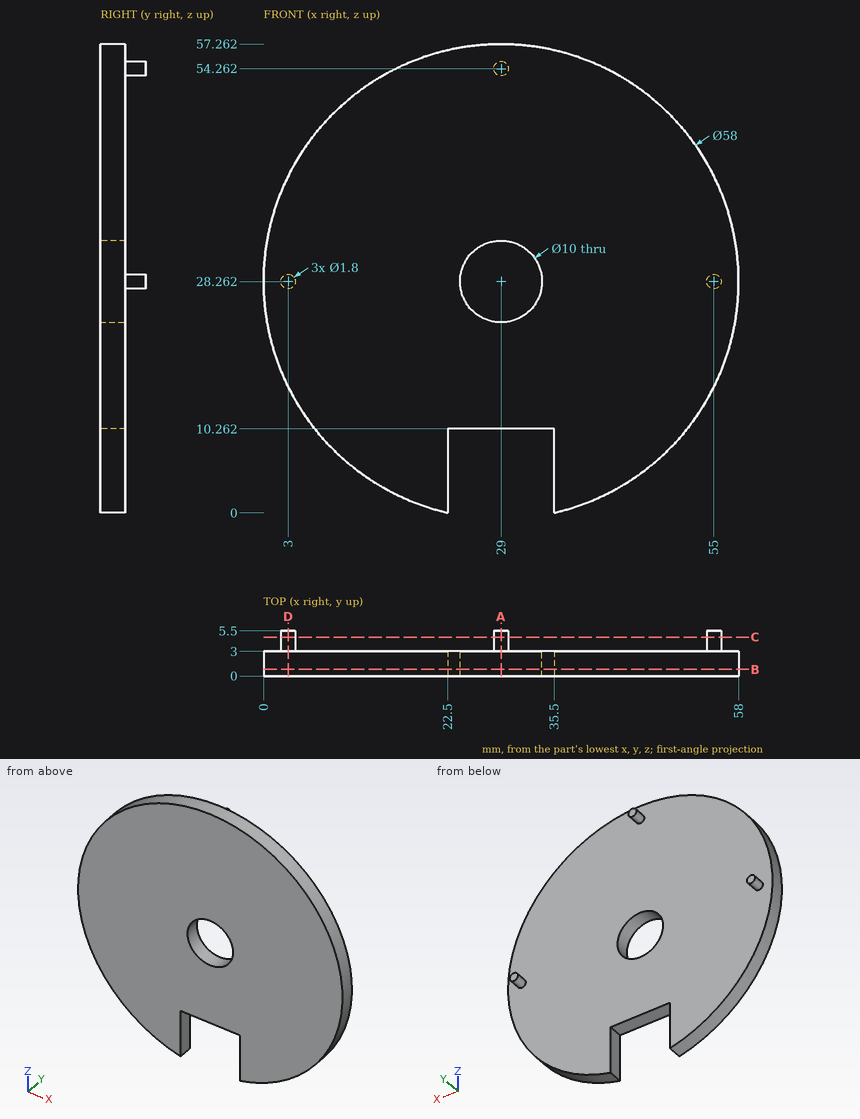
Part print with two shaded views. Sizes in mm from the minimum x, y, z corner. Coordinates: 2 decimals unless noted, no trailing zeros. Write each loop counter-clockwise with the first axis right and the second up, starting at its lowest first coordinate (ties: lowest second). Pieces come first, ordered by that corner, then holes.
1. Band-saw the part on D-D, the plane x = 3. Give the cut face in (y, z), and give its area (3 significant figures).
Answer block:
outline: (0, 15.42) - (3, 15.42) - (3, 27.36) - (5.5, 27.36) - (5.5, 29.16) - (3, 29.16) - (3, 41.11) - (0, 41.11) - close
area: 81.6 mm2
2. Band-saw the part on C-C, the plane y = 4.75. Give the cut face in (x, z).
Answer block:
outline: circle Ø1.8 at (3, 28.26); circle Ø1.8 at (29, 54.26); circle Ø1.8 at (55, 28.26)
3. Band-saw the part on B-B, the plane y = 0.8. Give the cut face in (x, z).
Answer block:
outline: (22.5, 0) - (22.5, 10.26) - (35.5, 10.26) - (35.5, 0) arc R29 ccw (long way) to start; hole circle Ø10 at (29, 28.26)
4. Band-saw the part on A-A, the plane x = 29. Give the cut face in (y, z), and give its area (4 significant figures).
Answer block:
outline: (0, 10.26) - (3, 10.26) - (3, 23.26) - (0, 23.26) - close; (0, 33.26) - (3, 33.26) - (3, 53.36) - (5.5, 53.36) - (5.5, 55.16) - (3, 55.16) - (3, 57.26) - (0, 57.26) - close
area: 115.5 mm2
5. Drill centre lines: probe 1 along Y at (x, z) = (55.5, 22.5); probe 2 along Z at (x, y) = (27, 0.75) (1 decimal); probe 3 along X at (y, z) = (1.2, 3). Where is each one in solid material? Low to high.
Answer block:
probe 1: y = 0 to 3
probe 2: z = 10.3 to 23.7, 32.8 to 57.2
probe 3: x = 14.76 to 22.5, 35.5 to 43.24
6. Drop flat-ended pins along their axis: pin 1 (1.5 mm diameter, centred on x = 30.5, y = 4, fed in from +Z); pin 2 (0.9 mm diameter, centred on x = 30, y = 1, fed in from -Z); pin 3 (8 mm diameter, centred on x = 29, z = 28.26, fed in from +Y); pin 4 (6 mm diameter, centred on x = 48, z = 47, fed in from +Y). Give the stop position or say it passes through.
Answer block:
pin 1: stops at z = 54.76
pin 2: stops at z = 10.26
pin 3: passes through
pin 4: stops at y = 3
